Source: CAD feature listing. Evaluate the final solid. Frame: model axes, mm. A direction names the side the tool comes from. Give positions to 0.01 mm unless a question says otherwise; leave off trailing zeros. Order: outer loops, then holes, each group sorted by start corner. A loop starts at its lowest first (then second) coordinate and runs counter-clockwise, first axis right, second up.
Autodesk Inventor part; units mm, degrees
ref_plane "YZ Plane" through (0, 0, 0) normal (1, 0, 0) x (0, 1, 0)
ref_plane "XZ Plane" through (0, 0, 0) normal (0, 1, 0) x (-1, 0, 0)
ref_plane "XY Plane" through (0, 0, 0) normal (0, 0, 1) x (1, 0, 0)
ref_plane "Work Plane1" through (0, 0, 9.525) normal (0, 0, 1) x (1, 0, 0)
sketch "Sketch1" plane through (0, 0, 0) normal (0, 0, 1) x (1, 0, 0)
  line L0 (0, 0) -> (6.35, 0)
  line L1 (6.35, 0) -> (6.35, 12.7)
  line L2 (6.35, 12.7) -> (25.4, 12.7)
  line L3 (25.4, 12.7) -> (25.4, 0)
  line L4 (25.4, 0) -> (31.75, 0)
  line L5 (31.75, 0) -> (31.75, 161.925)
  circle A0 centre (15.875, 25.4) radius 4.7816
  line L6 (-117.475, 161.925) -> (-117.475, 142.875)
  line L7 (0, 142.875) -> (0, 0)
  line L8 (-117.475, 142.875) -> (-117.475, 284.6917)
  line L9 (-54.61, 142.875) -> (-54.61, 111.125)
  line L10 (-54.61, 111.125) -> (-105.41, 142.875)
  line L11 (-117.475, 142.875) -> (-105.41, 142.875)
  line L12 (-54.61, 142.875) -> (0, 142.875)
  line L13 (-98.425, 284.6917) -> (-117.475, 284.6917)
  line L14 (-98.425, 265.5175) -> (-98.425, 256.0855)
  line L15 (-98.425, 238.125) -> (-98.425, 161.925)
  line L16 (31.75, 161.925) -> (-6.4592, 161.925)
  line L17 (-22.225, 161.925) -> (-98.425, 161.925)
  line L18 (-98.425, 284.6917) -> (-6.4592, 161.925)
  line L19 (-22.225, 161.925) -> (-98.425, 265.5175)
  line L20 (-98.425, 238.125) -> (-98.425, 256.0855)
  line L21 (31.75, 25.4) -> (31.75, 38.1)
  line L22 (31.75, 38.1) -> (0, 38.1) construction
  point P0 (-98.425, 263.525)
  point P1 (-6.35, 161.925)
  dimension "d0" = 6.35
  dimension "d1" = 12.7
  dimension "d2" = 19.05
  dimension "d3" = 6.35
  dimension "d4" = 161.925
  dimension "d5" = 9.5631
  dimension "d6" = 12.7
  dimension "d7" = 9.525
  dimension "d8" = 149.225
  dimension "d9" = 19.05
  dimension "d12" = 54.61
  dimension "d13" = 31.75
  dimension "d14" = 50.8
  dimension "d34" = 122.7667
  dimension "d37" = 19.05
  dimension "d38" = 19.05
  dimension "d39" = 76.2
  dimension "d40" = 76.2
  dimension "d41" = 19.05
  dimension "d50" = 0.5
  dimension "d51" = 12.7
  dimension "d61" = 12.7
sketch "Sketch2" plane through (0, 0, 9.525) normal (0, 0, 1) x (1, 0, 0)
  line L0 (-98.425, 298.45) -> (-117.475, 298.45)
  line L1 (-117.475, 284.6917) -> (-117.475, 142.875)
  circle A0 centre (-102.9208, 232.0925) radius 1.5875
  circle A1 centre (-113.03, 209.0801) radius 1.5875
  dimension "d24" = 3.175
  dimension "d25" = 14.5542
  dimension "d26" = 66.3575
  dimension "d27" = 3.175
  dimension "d29" = 89.3699
  dimension "d32" = 4.445
extrude "Extrusion4" add sketch "Sketch1" along normal blind 9.525
extrude "Extrusion5" cut sketch "Sketch2" against normal blind 9.525
fillet "Fillet2" radius 3.175 1 edges at (0, 142.875, 4.7625)
fillet "Fillet3" radius 3.175 1 edges at (-54.61, 142.875, 4.7625)
fillet "Fillet4" radius 3.175 1 edges at (-105.41, 142.875, 4.7625)
fillet "Fillet5" radius 3.175 6 edges at (-117.475, 284.6917, 4.7625) (-98.425, 284.6917, 4.7625) (-6.4592, 161.925, 4.7625) (-22.225, 161.925, 4.7625) (-98.425, 161.925, 4.7625) (-98.425, 265.5175, 4.7625)
sketch "Sketch4" plane through (0, 0, 9.525) normal (0, 0, 1) x (1, 0, 0)
  arc A0 (-97.4725, 283.4202) -> (-100.0136, 284.6917) centre (-100.0136, 281.5167) ccw
  line L0 (-100.0136, 284.6917) -> (-114.3, 284.6917)
  arc A1 (-114.3, 284.6917) -> (-117.475, 281.5167) centre (-114.3, 281.5167) ccw
  line L1 (-117.475, 281.5167) -> (-117.475, 142.875)
  line L2 (-117.475, 142.875) -> (-106.3206, 142.875)
  arc A2 (-104.6378, 142.3924) -> (-106.3206, 142.875) centre (-106.3206, 139.7) ccw
  line L3 (-104.6378, 142.3924) -> (-54.61, 111.125)
  line L4 (-54.61, 111.125) -> (-54.61, 139.7)
  arc A3 (-51.435, 142.875) -> (-54.61, 139.7) centre (-51.435, 139.7) ccw
  line L5 (-51.435, 142.875) -> (-3.175, 142.875)
  arc A4 (0, 139.7) -> (-3.175, 142.875) centre (-3.175, 139.7) ccw
  line L6 (0, 139.7) -> (0, 0)
  line L7 (0, 0) -> (6.35, 0)
  line L8 (6.35, 0) -> (6.35, 12.7)
  line L9 (6.35, 12.7) -> (25.4, 12.7)
  line L10 (25.4, 12.7) -> (25.4, 0)
  line L11 (25.4, 0) -> (31.75, 0)
  line L12 (31.75, 0) -> (31.75, 161.925)
  line L13 (31.75, 161.925) -> (-4.8706, 161.925)
  arc A5 (-7.4117, 163.1964) -> (-4.8706, 161.925) centre (-4.8706, 165.1) ccw
  line L14 (-7.4117, 163.1964) -> (-97.4725, 283.4202)
  line L15 (25.4, 0) -> (38.1, 0)
  line L16 (38.1, 0) -> (38.1, 25.4)
  line L17 (38.1, 25.4) -> (31.75, 25.4)
  dimension "d56" = 12.7
extrude "Extrusion7" add sketch "Sketch4" against normal blind 9.525 contours L17 L16 L15 L12
fillet "Fillet6" radius 3.175 4 edges at (38.1, 0, 4.7625) (25.4, 0, 4.7625) (6.35, 0, 4.7625) (0, 0, 4.7625)
fillet "Fillet7" radius 6.35 1 edges at (38.1, 25.4, 4.7625)
sketch "Sketch5" plane through (0, 0, 9.525) normal (0, 0, 1) x (1, 0, 0)
  arc A0 (38.1, 19.05) -> (31.75, 25.4) centre (31.75, 19.05) ccw
  line L0 (31.75, 25.4) -> (31.75, 161.925)
  line L1 (31.75, 161.925) -> (-4.8706, 161.925)
  arc A1 (-7.4117, 163.1964) -> (-4.8706, 161.925) centre (-4.8706, 165.1) ccw
  line L2 (-7.4117, 163.1964) -> (-97.4725, 283.4202)
  arc A2 (-97.4725, 283.4202) -> (-100.0136, 284.6917) centre (-100.0136, 281.5167) ccw
  line L3 (-100.0136, 284.6917) -> (-114.3, 284.6917)
  arc A3 (-114.3, 284.6917) -> (-117.475, 281.5167) centre (-114.3, 281.5167) ccw
  line L4 (-117.475, 281.5167) -> (-117.475, 142.875)
  line L5 (-117.475, 142.875) -> (-106.3206, 142.875)
  arc A4 (-104.6378, 142.3924) -> (-106.3206, 142.875) centre (-106.3206, 139.7) ccw
  line L6 (-104.6378, 142.3924) -> (-54.61, 111.125)
  line L7 (-54.61, 111.125) -> (-54.61, 139.7)
  arc A5 (-51.435, 142.875) -> (-54.61, 139.7) centre (-51.435, 139.7) ccw
  line L8 (-51.435, 142.875) -> (-3.175, 142.875)
  arc A6 (0, 139.7) -> (-3.175, 142.875) centre (-3.175, 139.7) ccw
  line L9 (0, 139.7) -> (0, 3.175)
  arc A7 (0, 3.175) -> (6.35, 3.175) centre (3.175, 3.175) ccw
  line L10 (6.35, 3.175) -> (6.35, 12.7)
  line L11 (6.35, 12.7) -> (25.4, 12.7)
  line L12 (25.4, 12.7) -> (25.4, 3.175)
  arc A8 (25.4, 3.175) -> (28.575, 0) centre (28.575, 3.175) ccw
  line L13 (28.575, 0) -> (34.925, 0)
  arc A9 (34.925, 0) -> (38.1, 3.175) centre (34.925, 3.175) ccw
  line L14 (38.1, 3.175) -> (38.1, 19.05)
  circle A10 centre (15.875, 25.4) radius 4.7816
  line L15 (-98.425, 165.1) -> (-98.425, 255.8428)
  arc A11 (-92.6924, 257.7241) -> (-98.425, 255.8428) centre (-95.25, 255.8428) ccw
  line L16 (-92.6924, 257.7241) -> (-25.9443, 166.9813)
  arc A12 (-28.5019, 161.925) -> (-25.9443, 166.9813) centre (-28.5019, 165.1) ccw
  line L17 (-28.5019, 161.925) -> (-95.25, 161.925)
  arc A13 (-98.425, 165.1) -> (-95.25, 161.925) centre (-95.25, 165.1) ccw
  circle A14 centre (-113.03, 209.0801) radius 1.5875
  circle A15 centre (-102.9208, 232.0925) radius 1.5875
  point P0 (0, 0)
properties part number "Right Climber Hook"
(1) Access query for faces 5 (the flat face through (16, 12.7, 5)), 6 (the flat face through (14, 161.925, 5)), 7 (the cylindrical face through (-25.691, 163.623, 4.829)), 8 (the flat face through (-112, 142.875, 5)). Directions: +Z, -Z, +X, -X, +Y, -Y. A direction counts if a zero-diameter tool reaches every point of the face in a straight line with its end or side. Return the directions, or none.
(2) Section B-B, the plane y = 65.5. Return loops of the section in (x, z) (3 decimals).
(3) Draft query along Y for faces 1 (the flat face through (-98.425, 211, 5)), 2 (the flat face through (6.35, 8, 5)), 3 (the flat face through (-107, 284.692, 5)), 4 (the cylindrical face through (14.84, 30.07, 4.7)). Return one class per face: +Y half, -Y half, draft (parallel to the pull), parting line (faces both ways), or undercut.
(4) Pin query (flat end, axial travel): pin 1 Ø4 at (x, z) = (-56.5, 2) entering from +Y; pin 2 Ø3 at (x, z) = (12.5, 2.5) entering from -Y; pin 3 Ø3 at (x, z) = (-68.5, 3.5) entering from +Y; pin 4 Ø1.5 at (x, y) = (22.5, 73.5) entering from -Z. Return the tip coordinate at first contact, or that it passes through.
(5) Line query: line 1 along Y through (x, z) = (-113.03, 5) (3 decimals); line 2 along X through (y, z) = (232.5, 7.5) (1 decimal); line 3 along X through (y, z) = (31, 8.75). Output: solid intervals per line, ascending.
(6) Section C-C, the plane z = 4. Count the separate pieces of the cut face and the enclosed holes in it, plus the area to 3 significant figures.
(7) Section A-A, the plane x = -48. Return loops of the section in (y, z) (3 decimals).
Checks:
1. face 5: +Z, -Z, -Y
1. face 6: +Z, -Z, +X, +Y
1. face 7: +Z, -Z
1. face 8: +Z, -Z, -X, -Y
2. outline: (0, 0) - (31.75, 0) - (31.75, 9.525) - (0, 9.525) - close
3. face 1: undercut
3. face 2: draft
3. face 3: +Y half
3. face 4: undercut
4. pin 1: stops at y = 231.4
4. pin 2: stops at y = 12.7
4. pin 3: stops at y = 246.75
4. pin 4: stops at z = 0
5. line 1: y = 142.875 to 207.493, 210.668 to 284.692
5. line 2: x = -117.5 to -104.5, -101.4 to -98.4, -74.1 to -59.3
5. line 3: x = 0 to 31.75
6. separate pieces: 1
6. enclosed holes: 4
6. area: 12,100 mm2
7. outline: (142.875, 0) - (161.925, 0) - (161.925, 9.525) - (142.875, 9.525) - close; (196.966, 0) - (217.379, 0) - (217.379, 9.525) - (196.966, 9.525) - close
